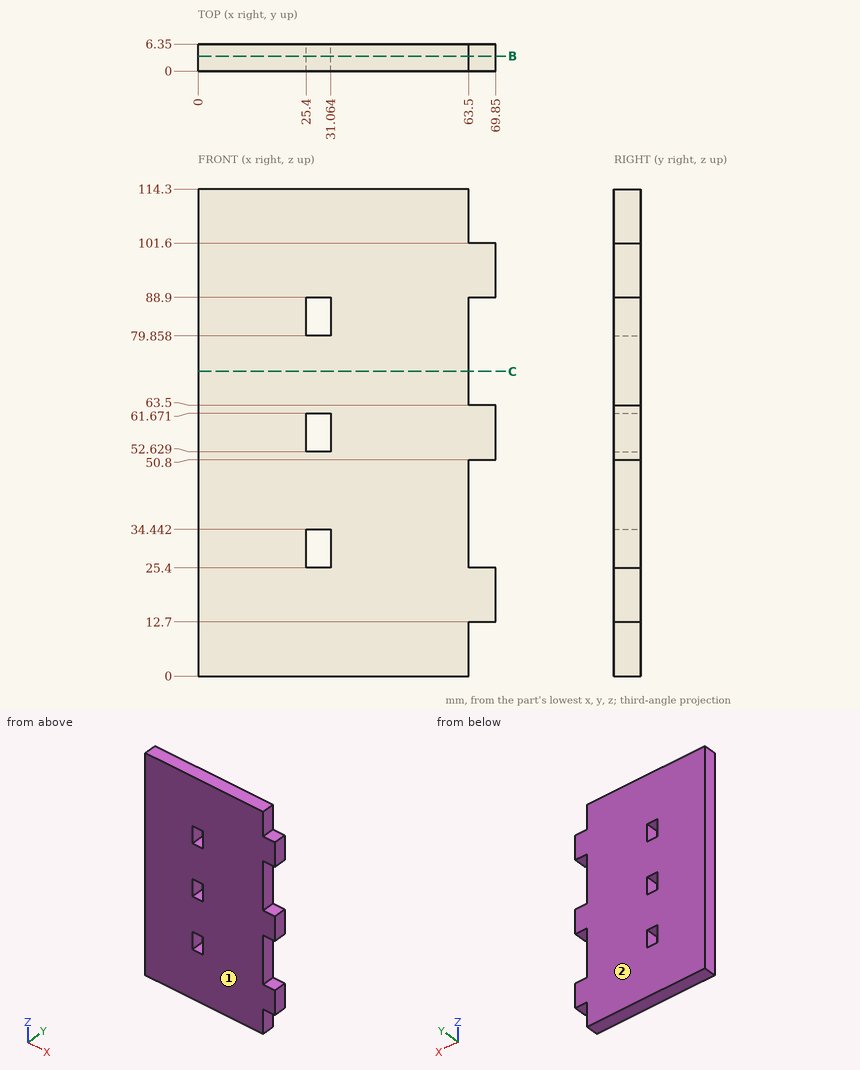
Answer from the drawing. Dimensions are ordinates in mm from the lowest x, y and z of the part. Give positions to 0.01 mm unless a question says otherwise; leave off trailing zeros. Write each loop counter-clockwise with the first axis right and the second up, starting at its lowest first coordinate (ties: lowest second). Pieces come first, ordered by that corner, then holes. Notation, with made-up numbers: (-37, 40.25) - (-31, 40.25) arc R14 ccw to (-31, 49.25) - close; hole circle Ø1 at (-3.5, -9). An arc over 180 degrees is marked (long way). One line per item, written item: value. Start each with the question number.
1. Find section B-B (y = 3.5). State how many separate pieces and enclosed holes the cut face has, then the cut area to 3 significant figures.
2. Consider probe 1 along Z at (x, y) = (65.5, 5); probe 2 along Z at (x, y) = (26.5, 1); probe 3 along X at (y, z) = (1.5, 83) (1 decimal). Determine where each line is inside the solid, lowest interval first.
3. Given pin 1 (1.9 mm diameter, centred on x = 65, y = 3, fed in from +Z), flat-ended and moving along its own axis, determine where the tip first touches the part or whether it passes through.
4. Find section C-C (z = 71.5). Write down the section's boundary in (x, y).
5. For a pull along Y with two mould halves and no side action, classify the marked faces 1 and 2 as +Y half, -Y half, draft (parallel to the pull), parting line (faces both ways), or undercut.
Geometry results:
1. separate pieces: 1
1. enclosed holes: 3
1. area: 7,350 mm2
2. probe 1: 12.7 to 25.4, 50.8 to 63.5, 88.9 to 101.6
2. probe 2: 0 to 25.4, 34.44 to 52.63, 61.67 to 79.86, 88.9 to 114.3
2. probe 3: 0 to 25.4, 31.1 to 63.5
3. pin 1: z = 101.6
4. outline: (0, 0) - (63.5, 0) - (63.5, 6.35) - (0, 6.35) - close
5. face 1: -Y half
5. face 2: +Y half
